CAD build for the part. Positions are in the model's coordinates, mm. A direction names the side the tool comes from. Round coordinates to 2 decimals unless told otherwise and drop trailing zeros. Loops run counter-clockwise (first coordinate to the right, second up) from the corner with the lowest first, then second, coordinate; pieces in that order, holes last. Notation, with made-up numbers: (85.25, 44) - (94.25, 44) arc R10 ccw to (94.25, 48) - close; hole circle Ø4 at (33.5, 32.25). An arc over 180 degrees is marked (long way). One line per question, with ' | ' between items.
```python
from build123d import *

# Parameters (mm, degrees)
F1_DEPTH = 5
F2_DEPTH = 10
F3_DEPTH = 3


with BuildPart() as f1:
    # F0 (on Top) → F1 (new body)
    with BuildSketch(Plane.XY):
        with BuildLine():
            Line((0.560707187, 3.4989949035), (0.560707187, 2.9471354652))
            ThreePointArc((0.560707187, 2.9471354652), (2.3110735126, 1.9128353874), (3, 0))
            ThreePointArc((3, 0), (-1.9287498107, -2.2978085577), (-0.5199494453, 2.9545985471))
            Line((-0.5199494453, 2.9545985471), (-0.5199494453, 3.4929679604))
            ThreePointArc((-0.5199494453, 3.4929679604), (-2.4505424978, 4.3861128404), (-3.5684511747, 6.1958579885))
            ThreePointArc((-3.5684511747, 6.1958579885), (-4.2026645539, 5.7844715098), (-4.7898990575, 5.3084241559))
            ThreePointArc((-4.7898990575, 5.3084241559), (-3.5543368281, 3.9728631878), (-3.1062443016, 2.2094715098))
            ThreePointArc((-3.1062443016, 2.2094715098), (-4.2581115343, -0.4705954297), (-6.9953231706, -1.4791733296))
            ThreePointArc((-6.9953231706, -1.4791733296), (-6.8000540915, -2.2094715098), (-6.5287715949, -2.9150714334))
            ThreePointArc((-6.5287715949, -2.9150714334), (-2.6133197512, -2.450072934), (-0.508854764, -5.7844715098))
            ThreePointArc((-0.508854764, -5.7844715098), (-0.5708860042, -6.4585748626), (-0.754896307, -7.1100373814))
            ThreePointArc((-0.754896307, -7.1100373814), (0, -7.15), (0.754896307, -7.1100373814))
            ThreePointArc((0.754896307, -7.1100373814), (2.0314976346, -2.7961166157), (6.5287715949, -2.9150714334))
            ThreePointArc((6.5287715949, -2.9150714334), (6.8000540915, -2.2094715098), (6.9953231706, -1.4791733296))
            ThreePointArc((6.9953231706, -1.4791733296), (3.2870322209, 1.0680215107), (4.7898990575, 5.3084241559))
            ThreePointArc((4.7898990575, 5.3084241559), (4.2026645539, 5.7844715098), (3.5684511747, 6.1958579885))
            ThreePointArc((3.5684511747, 6.1958579885), (2.4659186562, 4.3998225611), (0.560707187, 3.4989949035))
        make_face()
        with BuildLine():
            ThreePointArc((-0.5199494453, 2.9545985471), (0.0207176923, 2.999928462), (0.560707187, 2.9471354652))
            Line((0.560707187, 2.9471354652), (0.560707187, 3.4989949035))
            ThreePointArc((0.560707187, 3.4989949035), (0.0206004706, 3.4562476552), (-0.5199494453, 3.4929679604))
            Line((-0.5199494453, 3.4929679604), (-0.5199494453, 2.9545985471))
        make_face()
    extrude(amount=F1_DEPTH)

    # F0 (on Top) → F2 (join)
    with BuildSketch(Plane.XY):
        with BuildLine():
            ThreePointArc((0.560707187, 0.887754161), (0.9195766815, 0.5068320499), (1.05, 0))
            ThreePointArc((1.05, 0), (-0.527519233, -0.9078675337), (-0.5199494453, 0.9122239716))
            Line((-0.5199494453, 0.9122239716), (-0.5199494453, 2.9545985471))
            ThreePointArc((-0.5199494453, 2.9545985471), (-1.9287498107, -2.2978085577), (3, 0))
            ThreePointArc((3, 0), (2.3110735126, 1.9128353874), (0.560707187, 2.9471354652))
            Line((0.560707187, 2.9471354652), (0.560707187, 0.887754161))
        make_face()
        with BuildLine():
            ThreePointArc((-0.5199494453, 0.9122239716), (0.0237695453, 1.0497309221), (0.560707187, 0.887754161))
            Line((0.560707187, 0.887754161), (0.560707187, 2.9471354652))
            ThreePointArc((0.560707187, 2.9471354652), (0.0207176923, 2.999928462), (-0.5199494453, 2.9545985471))
            Line((-0.5199494453, 2.9545985471), (-0.5199494453, 0.9122239716))
        make_face()
    extrude(amount=F2_DEPTH)

    # F0 (on Top) → F3 (cut)
    with BuildSketch(Plane.XY):
        with BuildLine():
            ThreePointArc((-0.5199494453, 0.9122239716), (0.0237695453, 1.0497309221), (0.560707187, 0.887754161))
            Line((0.560707187, 0.887754161), (0.560707187, 2.9471354652))
            ThreePointArc((0.560707187, 2.9471354652), (0.0207176923, 2.999928462), (-0.5199494453, 2.9545985471))
            Line((-0.5199494453, 2.9545985471), (-0.5199494453, 0.9122239716))
        make_face()
        with BuildLine():
            ThreePointArc((-0.5199494453, 2.9545985471), (0.0207176923, 2.999928462), (0.560707187, 2.9471354652))
            Line((0.560707187, 2.9471354652), (0.560707187, 3.4989949035))
            ThreePointArc((0.560707187, 3.4989949035), (0.0206004706, 3.4562476552), (-0.5199494453, 3.4929679604))
            Line((-0.5199494453, 3.4929679604), (-0.5199494453, 2.9545985471))
        make_face()
    extrude(amount=F3_DEPTH, mode=Mode.SUBTRACT)


solid = f1.part
```
(1) Tool access for faces 4 (the face through (-1, 3, 5)), 5 (the face through (-6.803, -2.199, 2.465)), 6 (the face through (-0.52, 2, 1)): list every direction of +Z, -Z, +X, -X, +Y, -Y with a clear straight run to the whole face (end or side of a thin tool).
Results found:
face 4: +Z | face 5: +Z, -Z, -X, -Y | face 6: -Z, +Y
(2) Cut at B-B, the plane z = 0.5. Write the cut outline in (x, y).
Results found:
outline: (-7, -1.48) arc R7.15 ccw to (-6.53, -2.92) arc R3.69 cw to (-0.75, -7.11) arc R7.15 ccw to (0.75, -7.11) arc R3.69 cw to (6.53, -2.92) arc R7.15 ccw to (7, -1.48) arc R3.69 cw to (4.79, 5.31) arc R7.15 ccw to (3.57, 6.2) arc R3.69 cw to (0.56, 3.5) - (0.56, 0.89) arc R1.05 cw (long way) to (-0.52, 0.91) - (-0.52, 3.49) arc R3.69 cw to (-3.57, 6.2) arc R7.15 ccw to (-4.79, 5.31) arc R3.69 cw to start
(3) Drop flat-ended pins along their axis: P1, Ø5, axis at y = 3.5, z = 5.5, coming from the -X side; P2, Ø3, axis at y = 2, z = 1.5, coming from the -X side; P3, Ø2.5, axis at x = 0, y = 0, coming from the -Z side; P4, Ø1.5, axis at x = -2, z = 4.5, coming from the +Y side. Give the stop position or say it passes through.
Results found:
P1: stops at x = -4.79 | P2: stops at x = -3.53 | P3: stops at z = 0 | P4: stops at y = 4.68
(4) Probe L1, parallel to X at y = -2.5, z = 4.5; L2, parallel to Y at x = 0, z = 6; L3, parallel to Z at x = -2.75, y = -1.5. List the from-to ranges inside material, lowest first.
Results found:
L1: x = -6.7 to -5.89, -2.51 to 2.51, 5.89 to 6.7 | L2: y = -3 to -1.05, 1.05 to 3 | L3: z = 0 to 5
(5) Two-plate mould, pull along X, no slides. Class faces 1 (the face through (0, 2, 3)), 2 (the face through (0, -1.3, 10)), 3 (the face through (4.21, 5.78, 2.46)): released by +X, released by -X, zero draft, split by the parting line, or undercut.
Results found:
face 1: undercut | face 2: zero draft | face 3: released by +X
(6) Cut at C-C, the plane z = 5.25. Write the cut outline in (x, y), then the cut area to 3 significant figures.
Results found:
outline: circle Ø6 at (0, 0); hole circle Ø2.1 at (0, 0) | area: 24.8 mm²
(7) Cut at A-A, the plane x = 0. Write the cut outline in (y, z), then the cut area to 3 significant figures.
Results found:
outline: (-7.15, 0) - (-1.05, 0) - (-1.05, 10) - (-3, 10) - (-3, 5) - (-7.15, 5) - close; (1.05, 3) - (3.46, 3) - (3.46, 5) - (3, 5) - (3, 10) - (1.05, 10) - close | area: 54.8 mm²
(8) Cut at D-D, the plane y = 1.75. Write the cut outline in (x, z), then the cut area to 3 significant figures.
Results found:
outline: (-3.13, 0) - (-0.52, 0) - (-0.52, 3) - (0.56, 3) - (0.56, 0) - (3.13, 0) - (3.13, 5) - (2.44, 5) - (2.44, 10) - (-2.44, 10) - (-2.44, 5) - (-3.13, 5) - close | area: 52.5 mm²
